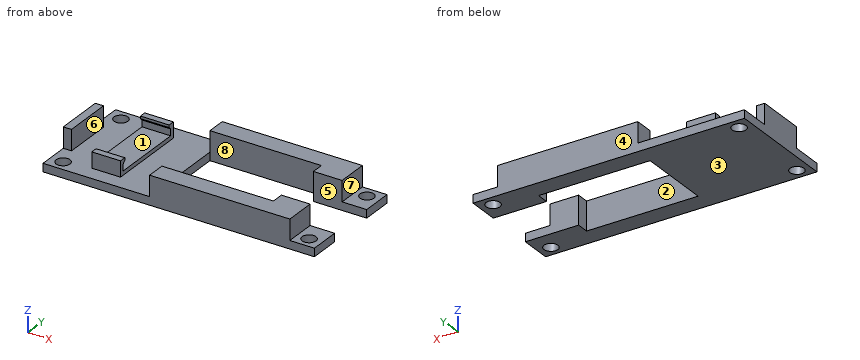
from build123d import *

# Parameters (mm, degrees)
SKETCH022_R  = 1.7
PAD005_DEPTH = 2
PAD006_DEPTH = 7
PAD007_DEPTH = 7
SKETCH025_W  = 2
SKETCH025_H  = 12
PAD008_DEPTH = 5


with BuildPart() as part:
    # Sketch022 → Pad005 (new body)
    with BuildSketch(Plane.XY):
        Polygon((-31.5, -13.6), (34.7, -13.6), (34.7, -6), (21.7, -6), (21.7, -9), (-5.5, -9), (-5.5, 9), (21.7, 9), (21.7, 6), (34.7, 6), (34.7, 13.6), (-31.5, 13.6), align=None)
        with Locations((31.6, 10.85)):
            Circle(SKETCH022_R, mode=Mode.SUBTRACT)
        with Locations((31.6, -10.85)):
            Circle(SKETCH022_R, mode=Mode.SUBTRACT)
        with Locations((-28.4, 10.85)):
            Circle(SKETCH022_R, mode=Mode.SUBTRACT)
        with Locations((-28.4, -10.85)):
            Circle(SKETCH022_R, mode=Mode.SUBTRACT)
    extrude(amount=PAD005_DEPTH)

    # Sketch023 → Pad006 (join)
    with BuildSketch(Plane.XY):
        Polygon((-5.5, 9), (-5.5, 13.6), (28.7, 13.6), (28.7, 6), (21.7, 6), (21.7, 9), align=None)
        Polygon((-5.5, -9), (-5.5, -13.6), (28.7, -13.6), (28.7, -6), (21.7, -6), (21.7, -9), align=None)
    extrude(amount=PAD006_DEPTH)

    # Sketch024 → Pad007 (join)
    with BuildSketch(Plane.YZ.offset(-15)):
        Polygon((9.9, 0), (9.9, 5.8), (8.3, 5.8), (8.3, 5.2), (8.9, 4.6), (8.9, 3), (-8.9, 3), (-8.9, 4.6), (-8.3, 5.2), (-8.3, 5.8), (-9.9, 5.8), (-9.9, 0), align=None)
    extrude(amount=-PAD007_DEPTH)

    # Sketch025 (on Face4 of Pad007) → Pad008 (join)
    with BuildSketch(Plane.XY.offset(2)):
        with Locations((-30.5, 0)):
            Rectangle(SKETCH025_W, SKETCH025_H)
    extrude(amount=PAD008_DEPTH)


solid = part.part
The listing builds one solid part. Answer for the finished solid, in the listing's coordinates (mm). Face numbers are marked on the shaded views. A direction names the side the tool comes from. Give positions to 0.01 mm unless a question says otherwise; leave off trailing zeros. Write each loop counter-clockwise with the first axis right and the second up, starting at its lowest first coordinate (ties: lowest second). Pieces come first, ordered by that corner, then holes.
1) For a pull along Y with two mould halves and no side action, classify the marked faces 1, 2, 3 and 4 as pulls with the +Y half, pulls with the -Y half, needs draft (parallel to the pull), parting line crosses it, or undercut.
2) Section D-D (x = 4) is taken. Write down the section's boundary in (y, z).
3) Section C-C (z = 1) is taken. Write down the section's boundary in (x, y), and give its area (3 significant figures).
4) Section A-A (x = -28.4) is taken. Write down the section's boundary in (y, z), and give its area (3 significant figures).
5) Find the intervals of material crossed by L1, parallel to Y at x = -28.4, z = 1.55; L2, parallel to Y at x = 31.6, z = 1.5; L3, parallel to X at y = 2.25, z = 2.25, in increasing order.
6) Section B-B (y = 10.85) is taken. Write down the section's boundary in (x, z), and give its area (3 significant figures).
7) Given P1, Ø6, axis at x = -6.5, y = 2.5, coming from the +Z side; P2, Ø2.5, axis at y = -9, z = 4.5, coming from the +X side; P3, Ø5, axis at x = 26.5, y = 2.5, coming from the -Z side; P4, Ø2.5, axis at y = -7, z = 4, coming from the -X side, each flat-ended and moving along its own axis, determine where each tip first touches the part or whether it passes through.
8) A tool of negligible diameter and unlimited length cuts with its end or side. For the marked faces 5, 6, 7 and 8, from which of +Z, -Z, +X, -X, +Y, -Y can it reach the whole face along a straight path? Write none if from no direction.
Response:
1. face 1: undercut
1. face 2: undercut
1. face 3: needs draft
1. face 4: pulls with the +Y half
2. outline: (-13.6, 0) - (-9, 0) - (-9, 7) - (-13.6, 7) - close; (9, 0) - (13.6, 0) - (13.6, 7) - (9, 7) - close
3. outline: (-31.5, -13.6) - (34.7, -13.6) - (34.7, -6) - (21.7, -6) - (21.7, -9) - (-5.5, -9) - (-5.5, 9) - (21.7, 9) - (21.7, 6) - (34.7, 6) - (34.7, 13.6) - (-31.5, 13.6) - close; hole circle Ø3.4 at (-28.4, -10.85); hole circle Ø3.4 at (-28.4, 10.85); hole circle Ø3.4 at (31.6, -10.85); hole circle Ø3.4 at (31.6, 10.85)
3. area: 1,120 mm2
4. outline: (-13.6, 0) - (-12.55, 0) - (-12.55, 2) - (-13.6, 2) - close; (-9.15, 0) - (9.15, 0) - (9.15, 2) - (-9.15, 2) - close; (12.55, 0) - (13.6, 0) - (13.6, 2) - (12.55, 2) - close
4. area: 40.8 mm2
5. L1: y = -13.6 to -12.55, -9.15 to 9.15, 12.55 to 13.6
5. L2: y = -13.6 to -12.55, -9.15 to -6, 6 to 9.15, 12.55 to 13.6
5. L3: x = -31.5 to -29.5, -22 to -15
6. outline: (-31.5, 0) - (-30.1, 0) - (-30.1, 2) - (-31.5, 2) - close; (-26.7, 0) - (29.9, 0) - (29.9, 2) - (28.7, 2) - (28.7, 7) - (-5.5, 7) - (-5.5, 2) - (-26.7, 2) - close; (33.3, 0) - (34.7, 0) - (34.7, 2) - (33.3, 2) - close
6. area: 290 mm2
7. P1: stops at z = 2
7. P2: stops at x = 28.7
7. P3: passes through
7. P4: stops at x = -31.5
8. face 5: +Z, -Z, +X
8. face 6: +Z, +Y, -Y
8. face 7: +Z, +X, +Y, -Y
8. face 8: +Z, -Z
